Model file for the job. Use its own axes, mm. Give positions to 0.01 mm unless a question says otherwise; leave off trailing zeros. Order: outer loops, then holes, each group sorted by start corner. A loop starts at its lowest first (then second) coordinate and runs counter-clockwise, first axis right, second up. Notation, with made-up numbers: (-35.75, -4.75) - (-13.75, -4.75) arc R29 ccw to (-13.75, 23.25) - close; hole circle Ø6 at (63, -14). An arc over 180 degrees is marked (long way). Return JSON: item names as keys, results as strings. Group by question number.
from build123d import *

# Parameters (mm, degrees)
SKETCH1_W           = 228
SKETCH1_H           = 217
SKETCH1_R           = 2.5
SKETCH1_R_2         = 6.75
SKETCH1_R_3         = 10
SKETCH1_R_4         = 1.5
SKETCH1_W_2         = 7
SKETCH1_H_2         = 5
BOSS_EXTRUDE1_DEPTH = 1
SKETCH5_R           = 1.25
CUT_EXTRUDE3_DEPTH  = 315.760226204
FILLET1_R           = 0.5


with BuildPart() as part:
    # Sketch1 → Boss-Extrude1 (new body)
    with BuildSketch(Plane(origin=(0, 0, 0), x_dir=(0, 0, -1), z_dir=(1, 0, 0))):
        with Locations((114, 108.5)):
            Rectangle(SKETCH1_W, SKETCH1_H)
        with Locations((13, 10.85)):
            Circle(SKETCH1_R, mode=Mode.SUBTRACT)
        with Locations((13, 211.15)):
            Circle(SKETCH1_R, mode=Mode.SUBTRACT)
        with Locations((67.5, 14)):
            Circle(SKETCH1_R_2, mode=Mode.SUBTRACT)
        with Locations((216, 10.85)):
            Circle(SKETCH1_R, mode=Mode.SUBTRACT)
        with Locations((216, 211.15)):
            Circle(SKETCH1_R, mode=Mode.SUBTRACT)
        with Locations((60.05, 149)):
            Circle(SKETCH1_R_3, mode=Mode.SUBTRACT)
        with Locations((77, 14)):
            Circle(SKETCH1_R_4, mode=Mode.SUBTRACT)
        with Locations((58, 14)):
            Circle(SKETCH1_R_4, mode=Mode.SUBTRACT)
        with Locations((147.63, 12.5)):
            Rectangle(SKETCH1_W_2, SKETCH1_H_2, mode=Mode.SUBTRACT)
        with Locations((147.63, 163.5)):
            Rectangle(SKETCH1_W_2, SKETCH1_H_2, mode=Mode.SUBTRACT)
        with BuildLine():
            Line((78.5, 41.2), (77.427738917, 41.2))
            ThreePointArc((77.427738917, 41.2), (66.898913138, 49.981918382), (57.5, 40))
            ThreePointArc((57.5, 40), (66.898913138, 30.018081618), (77.427738917, 38.8))
            Line((77.427738917, 38.8), (78.5, 38.8))
            Line((78.5, 38.8), (78.5, 41.2))
        make_face(mode=Mode.SUBTRACT)
    extrude(amount=BOSS_EXTRUDE1_DEPTH)

    # Sketch5 → Cut-Extrude3 (cut, through all)
    with BuildSketch(Plane(origin=(1, 0, 0), x_dir=(0, 0, -1), z_dir=(1, 0, 0))):
        with Locations((145.013883476, 165.116116524)):
            Circle(SKETCH5_R)
        with Locations((150.246116524, 165.116116524)):
            Circle(SKETCH5_R)
        with Locations((145.013883476, 161.883883476)):
            Circle(SKETCH5_R)
        with Locations((150.246116524, 161.883883476)):
            Circle(SKETCH5_R)
        with Locations((150.246116524, 14.116116524)):
            Circle(SKETCH5_R)
        with Locations((150.246116524, 10.883883476)):
            Circle(SKETCH5_R)
        with Locations((145.013883476, 10.883883476)):
            Circle(SKETCH5_R)
        with Locations((145.013883476, 14.116116524)):
            Circle(SKETCH5_R)
        with BuildLine():
            Line((34.05, 110.25), (38.05, 110.25))
            ThreePointArc((38.05, 110.25), (39.85, 103.25), (38.05, 96.25))
            Line((38.05, 96.25), (34.05, 96.25))
            ThreePointArc((34.05, 96.25), (29.85, 103.25), (34.05, 110.25))
        make_face()
        with BuildLine():
            Line((31.44, 35.265), (39.44, 35.265))
            ThreePointArc((39.44, 35.265), (40.147106781, 34.972106781), (40.44, 34.265))
            Line((40.44, 34.265), (40.44, 24.265))
            ThreePointArc((40.44, 24.265), (40.147106781, 23.557893219), (39.44, 23.265))
            Line((39.44, 23.265), (31.44, 23.265))
            ThreePointArc((31.44, 23.265), (30.732893219, 23.557893219), (30.44, 24.265))
            Line((30.44, 24.265), (30.44, 34.265))
            ThreePointArc((30.44, 34.265), (30.732893219, 34.972106781), (31.44, 35.265))
        make_face()
    extrude(amount=-CUT_EXTRUDE3_DEPTH, mode=Mode.SUBTRACT)

    # Fillet1
    fillet1_edges = [part.edges().sort_by_distance(p)[0] for p in [
        (0.5, 0, -228),
        (0.5, 0, 0),
        (0.5, 217, 0),
        (0.5, 217, -228),
    ]]
    fillet(fillet1_edges, radius=FILLET1_R)


solid = part.part
(1) Slice it at A-A (y = 106.5). Give the cut face in (x, z), and give its area (3 significant figures).
(2) Drill centre lines: L1, parallel to Y at x = 0.65, z = -13; L2, parallel to Z at x = 0.65, y = 211.15; L3, parallel to Z at x = 0.8, y = 28.5. Where is each one in solid material? Low to high.
(3) Slice it at C-C (z = -67.5). Give the cut face in (x, y).
(4) Drop a flat-ended pin along its axis: pin 1 Ø8 at (y, z) = (14, -67.5) entering from -X. Give the stop position or say it passes through.
(5) Slice it at B-B (x = 0.8). State how many separate pieces and enclosed holes the cut face has, and give its area (3 significant figures).
Result set:
{
 "1": {"outline": "(0, -228) - (1, -228) - (1, -39.48) - (0, -39.48) - close; (0, -30.55) - (1, -30.55) - (1, 0) - (0, 0) - close", "area": "219 mm²"},
 "2": {"L1": "y = 0 to 8.35, 13.35 to 208.65, 213.65 to 217", "L2": "z = -228 to -218.5, -213.5 to -15.5, -10.5 to 0", "L3": "z = -228 to -40.44, -30.44 to 0"},
 "3": {"outline": "(0, 0) - (1, 0) - (1, 7.25) - (0, 7.25) - close; (0, 20.75) - (1, 20.75) - (1, 30) - (0, 30) - close; (0, 50) - (1, 50) - (1, 142.33) - (0, 142.33) - close; (0, 155.67) - (1, 155.67) - (1, 217) - (0, 217) - close"},
 "4": {"pin 1": "passes through"},
 "5": {"separate pieces": "1", "enclosed holes": "13", "area": "48,300 mm²"}
}
